```python
from build123d import *

# Parameters (mm, degrees)
SKETCH1_W               = 113
SKETCH1_H               = 175.618176042
BOSS_EXTRUDE1_DEPTH     = 0.5
SKETCH2_R               = 4
SKETCH2_R_2             = 2
BOSS_EXTRUDE2_DEPTH     = 11
CUT_EXTRUDE1_DEPTH      = 3
SKETCH4_W               = 5
SKETCH4_H               = 8
BOSS_EXTRUDE3_DEPTH     = 8
CUT_EXTRUDE2_REACH      = 194.244
SKETCH5_R               = 1.75
CUT_EXTRUDE3_DEPTH      = 2.5
MIRROR2_COPY_1_SKETCH_W = 5
MIRROR2_COPY_1_SKETCH_H = 8
MIRROR2_COPY_1_DEPTH    = 8
MIRROR2_COPY_2_REACH    = 194.244
MIRROR2_COPY_2_SKETCH_R = 1.75
MIRROR2_COPY_3_DEPTH    = 2.5


with BuildPart() as part:
    # Sketch1 → Boss-Extrude1 (new body)
    with BuildSketch(Plane.XY):
        with Locations((52.5, 73.5)):
            Rectangle(SKETCH1_W, SKETCH1_H)
    extrude(amount=BOSS_EXTRUDE1_DEPTH)

    # Sketch2 → Boss-Extrude2 (add)
    with BuildSketch(Plane(origin=(0, 0, 0), x_dir=(-1, 0, 0), z_dir=(0, 0, -1))):
        with Locations(Location((-5.6, 120.15, 0), (0, 0, 180))):
            Circle(SKETCH2_R)
        with Locations(Location((-5.6, 120.15, 0), (0, 0, 180))):
            Circle(SKETCH2_R_2, mode=Mode.SUBTRACT)
        with Locations(Location((-5.6, 26.85, 0), (0, 0, 180))):
            Circle(SKETCH2_R)
        with Locations(Location((-5.6, 26.85, 0), (0, 0, 180))):
            Circle(SKETCH2_R_2, mode=Mode.SUBTRACT)
        with Locations(Location((-99.4, 26.85, 0), (0, 0, 180))):
            Circle(SKETCH2_R)
        with Locations(Location((-99.4, 26.85, 0), (0, 0, 180))):
            Circle(SKETCH2_R_2, mode=Mode.SUBTRACT)
        with Locations(Location((-99.4, 120.15, 0), (0, 0, 180))):
            Circle(SKETCH2_R)
        with Locations(Location((-99.4, 120.15, 0), (0, 0, 180))):
            Circle(SKETCH2_R_2, mode=Mode.SUBTRACT)
    extrude(amount=BOSS_EXTRUDE2_DEPTH)

    # Sketch3 → Cut-Extrude1 (cut)
    with BuildSketch(Plane(origin=(0, 0, 0), x_dir=(-1, 0, 0), z_dir=(0, 0, -1))):
        Polygon((-101.132050808, 123.15), (-97.667949192, 123.15), (-95.935898385, 120.15), (-97.667949192, 117.15), (-101.132050808, 117.15), (-102.864101615, 120.15), align=None)
        with BuildLine():
            Line((-95.935898385, 120.15), (-97.667949192, 117.15))
            Line((-97.667949192, 117.15), (-96.754248689, 117.15))
            ThreePointArc((-96.754248689, 117.15), (-95.754248689, 118.504248689), (-95.4, 120.15))
            ThreePointArc((-95.4, 120.15), (-95.754248689, 121.795751311), (-96.754248689, 123.15))
            Line((-96.754248689, 123.15), (-97.667949192, 123.15))
            Line((-97.667949192, 123.15), (-95.935898385, 120.15))
        make_face()
        Polygon((-3.867949192, 123.15), (-7.332050808, 123.15), (-9.064101615, 120.15), (-7.332050808, 117.15), (-3.867949192, 117.15), (-2.135898385, 120.15), align=None)
        with BuildLine():
            Line((-9.064101615, 120.15), (-7.332050808, 123.15))
            Line((-7.332050808, 123.15), (-8.245751311, 123.15))
            ThreePointArc((-8.245751311, 123.15), (-9.6, 120.15), (-8.245751311, 117.15))
            Line((-8.245751311, 117.15), (-7.332050808, 117.15))
            Line((-7.332050808, 117.15), (-9.064101615, 120.15))
        make_face()
        Polygon((-3.867949192, 23.85), (-7.332050808, 23.85), (-9.064101615, 26.85), (-7.332050808, 29.85), (-3.867949192, 29.85), (-2.135898385, 26.85), align=None)
        with BuildLine():
            Line((-9.064101615, 26.85), (-7.332050808, 29.85))
            Line((-7.332050808, 29.85), (-8.245751311, 29.85))
            ThreePointArc((-8.245751311, 29.85), (-9.6, 26.85), (-8.245751311, 23.85))
            Line((-8.245751311, 23.85), (-7.332050808, 23.85))
            Line((-7.332050808, 23.85), (-9.064101615, 26.85))
        make_face()
        Polygon((-101.132050808, 23.85), (-97.667949192, 23.85), (-95.935898385, 26.85), (-97.667949192, 29.85), (-101.132050808, 29.85), (-102.864101615, 26.85), align=None)
        with BuildLine():
            Line((-95.935898385, 26.85), (-97.667949192, 23.85))
            Line((-97.667949192, 23.85), (-96.754248689, 23.85))
            ThreePointArc((-96.754248689, 23.85), (-95.754248689, 25.204248689), (-95.4, 26.85))
            ThreePointArc((-95.4, 26.85), (-95.754248689, 28.495751311), (-96.754248689, 29.85))
            Line((-96.754248689, 29.85), (-97.667949192, 29.85))
            Line((-97.667949192, 29.85), (-95.935898385, 26.85))
        make_face()
    extrude(amount=CUT_EXTRUDE1_DEPTH, mode=Mode.SUBTRACT)

    # Sketch4 → Boss-Extrude3 (add)
    with BuildSketch(Plane(origin=(0, 0, 0), x_dir=(-1, 0, 0), z_dir=(0, 0, -1))):
        with Locations((-102.5, 18.5)):
            Rectangle(SKETCH4_W, SKETCH4_H)
        with BuildLine():
            add(Edge.make_bspline(
                [(-105, 22.5), (-105, 25.54291505), (-104.360830865, 28.066908547), (-101.849562653, 30.012221183)],
                knots=[0, 0, 0, 0, 1, 1, 1, 1], degree=3))
            Line((-105, 22.5), (-100, 22.5))
            Line((-100, 22.5), (-100, 22.895256013))
            ThreePointArc((-100, 22.895256013), (-103.271402382, 25.843896824), (-101.849562653, 30.012221183))
        make_face()
    boss_extrude3 = extrude(amount=BOSS_EXTRUDE3_DEPTH)

    # Sketch5 → Cut-Extrude2 (cut, up to next)
    with BuildSketch(Plane.ZY.offset(-100), mode=Mode.PRIVATE) as cut_extrude2_sk1:
        with Locations((-3.896353455, 18.5)):
            Circle(SKETCH5_R)
    cut_extrude2_tool1 = extrude(cut_extrude2_sk1.sketch, amount=-CUT_EXTRUDE2_REACH, mode=Mode.PRIVATE) & part.part
    cut_extrude2 = cut_extrude2_tool1.solids().sort_by_distance((100, 18.5, -3.896353))[0]
    add(cut_extrude2, mode=Mode.SUBTRACT)

    # Sketch6 → Cut-Extrude3 (cut)
    with BuildSketch(Plane.ZY.offset(-100)):
        Polygon((-3.896353455, 21.964101615), (-6.896353455, 20.232050808), (-6.896353455, 16.767949192), (-3.896353455, 15.035898385), (-0.896353455, 16.767949192), (-0.896353455, 20.232050808), align=None)
    cut_extrude3 = extrude(amount=-CUT_EXTRUDE3_DEPTH, mode=Mode.SUBTRACT)

    # Mirror1: Boss-Extrude3, Cut-Extrude2, Cut-Extrude3 across plane
    add(boss_extrude3.mirror(Plane.ZY.offset(-52.5)))
    add(cut_extrude2.mirror(Plane.ZY.offset(-52.5)), mode=Mode.SUBTRACT)
    add(cut_extrude3.mirror(Plane.ZY.offset(-52.5)), mode=Mode.SUBTRACT)

    # Mirror2: Boss-Extrude3, Cut-Extrude2, Cut-Extrude3 across plane
    add(boss_extrude3.mirror(Plane(origin=(0, 73.5, 0), x_dir=(0, 0, 1), z_dir=(0, -1, 0))))
    add(cut_extrude2.mirror(Plane(origin=(0, 73.5, 0), x_dir=(0, 0, 1), z_dir=(0, -1, 0))), mode=Mode.SUBTRACT)
    add(cut_extrude3.mirror(Plane(origin=(0, 73.5, 0), x_dir=(0, 0, 1), z_dir=(0, -1, 0))), mode=Mode.SUBTRACT)

    # Mirror2 copy 1 sketch → Mirror2 copy 1 (add)
    with BuildSketch(Plane(origin=(105, 147, 0), x_dir=(1, 0, 0), z_dir=(0, 0, -1))):
        with Locations((-102.5, 18.5)):
            Rectangle(MIRROR2_COPY_1_SKETCH_W, MIRROR2_COPY_1_SKETCH_H)
        with BuildLine():
            add(Edge.make_bspline(
                [(-105, 22.5), (-105, 25.54291505), (-104.360830865, 28.066908547), (-101.849562653, 30.012221183)],
                knots=[0, 0, 0, 0, 1, 1, 1, 1], degree=3))
            Line((-105, 22.5), (-100, 22.5))
            Line((-100, 22.5), (-100, 22.895256013))
            ThreePointArc((-100, 22.895256013), (-103.271402382, 25.843896824), (-101.849562653, 30.012221183))
        make_face()
    extrude(amount=MIRROR2_COPY_1_DEPTH)

    # Mirror2 copy 2 sketch → Mirror2 copy 2 (cut, up to next)
    with BuildSketch(Plane(origin=(5, 147, 0), x_dir=(0, 0, 1), z_dir=(1, 0, 0)), mode=Mode.PRIVATE) as mirror2_copy_2_sk1:
        with Locations((-3.896353455, 18.5)):
            Circle(MIRROR2_COPY_2_SKETCH_R)
    mirror2_copy_2_tool1 = extrude(mirror2_copy_2_sk1.sketch, amount=-MIRROR2_COPY_2_REACH, mode=Mode.PRIVATE) & part.part
    add(mirror2_copy_2_tool1.solids().sort_by_distance((5, 128.5, -3.896353))[0], mode=Mode.SUBTRACT)

    # Mirror2 copy 3 sketch → Mirror2 copy 3 (cut)
    with BuildSketch(Plane(origin=(5, 147, 0), x_dir=(0, 0, 1), z_dir=(1, 0, 0))):
        Polygon((-3.896353455, 21.964101615), (-6.896353455, 20.232050808), (-6.896353455, 16.767949192), (-3.896353455, 15.035898385), (-0.896353455, 16.767949192), (-0.896353455, 20.232050808), align=None)
    extrude(amount=-MIRROR2_COPY_3_DEPTH, mode=Mode.SUBTRACT)


solid = part.part
```
For this review, take the finished solid that the model builds, in its own axes (mm). A direction names the side the tool comes from. Coordinates: 2 decimals unless noted, no trailing zeros. Loops run counter-clockwise (first coordinate to the right, second up) from the corner with the lowest first, then second, coordinate; pieces in that order, holes last.
1. Add section B-B, the plane x = 19. Give the boundary of the cut face in (y, z).
2. For line 1 (X direction, y = 26.85, z = -8.5); line 2 (Y direction, x = 5.6, z = -6.25); line 3 (X direction, y = 125, z = -7.75), list the stretches that pass through material, from the lowest coordinate up.
3. Insertion check: P1, Ø1.5, axis at x = 2.5, z = -2.5, coming from the +Y side; P2, Ø2.5, axis at y = 19, z = -5, coming from the -X side; P3, Ø6.5, axis at y = 128.5, z = -4.5, coming from the +X side. Each pin has a flat end and moves straight along its axis. Give the tip position at first contact, or say it passes through.
4. Add section C-C, the plane y = 59.5. Give the boundary of the cut face in (x, z), then the cut area to 3 significant figures.
5. Mouldability with a two-part tool opening along Y and no side actions: class faces 1 (the flat face through (2, 14.5, -4)), 2 (the flat face through (6, 118, -11)), 3 (the flat face through (97, 121, -3)) as +Y half, -Y half, draft (parallel to the pull), parting line (faces both ways), or undercut.
6. For faces 4 (the cylindrical face through (6.523, 28.624, -6.944)), 5 (the flat face through (105, 129, -6)), 6 (the flat face through (8, 121, -3)), 7 (the flat face through (0, 18, -6)), list the 3-axis set-ups (+Z, -Z, +X, -X, +Y, -Y) from which the entire face can be reached by the end or side of a thin tool; tool diameter is ignored.
7. Add section A-A, the plane y = 128.5. Give the boundary of the cut face in (x, z), then the cut area to 3 significant figures.
Result:
1. outline: (-14.31, 0) - (161.31, 0) - (161.31, 0.5) - (-14.31, 0.5) - close
2. line 1: x = 1.6 to 3.6, 7.6 to 9.6, 95.4 to 97.4, 101.4 to 103.4
2. line 2: y = 22.85 to 24.85, 28.85 to 30.85, 116.15 to 118.15, 122.15 to 124.15
2. line 3: x = 0 to 5, 100 to 105
3. P1: stops at y = 132.5
3. P2: stops at x = 0
3. P3: stops at x = 105
4. outline: (-4, 0) - (109, 0) - (109, 0.5) - (-4, 0.5) - close
4. area: 56.5 mm2
5. face 1: -Y half
5. face 2: draft
5. face 3: undercut
6. face 4: -Z
6. face 5: -Z, +X, +Y, -Y
6. face 6: none
6. face 7: -Z, -X, +Y, -Y
7. outline: (-4, 0) - (0, 0) - (0, -2.15) - (2.5, -2.15) - (2.5, -0.9) - (5, -0.9) - (5, 0) - (100, 0) - (100, -0.9) - (102.5, -0.9) - (102.5, -2.15) - (105, -2.15) - (105, 0) - (109, 0) - (109, 0.5) - (-4, 0.5) - close; (0, -8) - (5, -8) - (5, -6.9) - (2.5, -6.9) - (2.5, -5.65) - (0, -5.65) - close; (100, -8) - (105, -8) - (105, -5.65) - (102.5, -5.65) - (102.5, -6.9) - (100, -6.9) - close
7. area: 89.0 mm2
